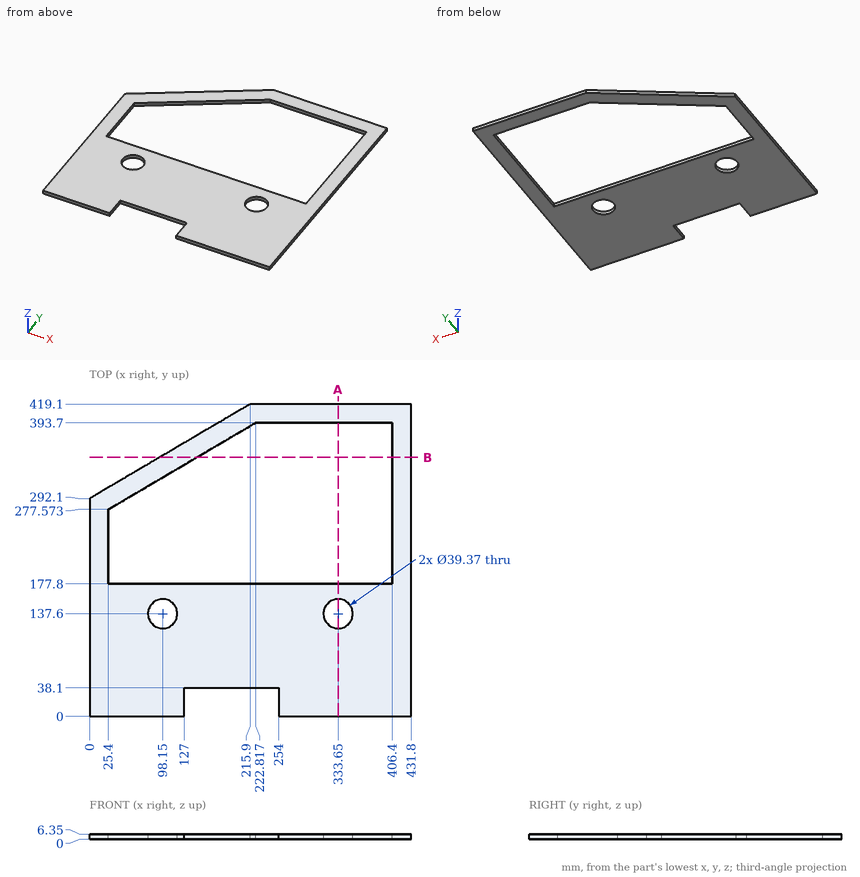
Input: dimensioned drawing with shaded views. Units: mm. Origin: part minimum x, y, z. Give positions to 0.01 mm unless a question says otherwise; leave off trailing zeros. Write each loop counter-clockwise with the first axis right and the second up, starting at its lowest first coordinate (ties: lowest second). Pieces come first, ordered by that corner, then holes.
1. Section query B-B (y = 347.5). Return the cut outline in (x, z).
2. Material intervals for line 1 along Y through (x, z) = (280.5, 1); line 2 along Y through (x, z) = (81.5, 3.75) (1 decimal); line 3 along X through (y, z) = (197.5, 2), sorted ascending.
3. First-contact query: pin 1 (2 mm diameter, centred on y = 313.5, z = 5.5, fed in from -X); pin 2 (23.5 mm diameter, centred on x = 333.65, y = 137.6, fed in from +Z). Flat tips, straight axial feed; report the tip coordinate or a pass-through.
4. Section query A-A (x = 333.65). Count the separate pieces of the cut face and the enclosed holes in it, then the cut area to 3 significant figures.
Output values:
1. outline: (94.18, 0) - (144.28, 0) - (144.28, 6.35) - (94.18, 6.35) - close; (406.4, 0) - (431.8, 0) - (431.8, 6.35) - (406.4, 6.35) - close
2. line 1: y = 0 to 177.8, 393.7 to 419.1
2. line 2: y = 0 to 127.1, 148.1 to 177.8, 310.6 to 340
2. line 3: x = 0 to 25.4, 406.4 to 431.8
3. pin 1: stops at x = 34.68
3. pin 2: passes through
4. separate pieces: 3
4. enclosed holes: 0
4. area: 1,040 mm2
